Build history of the part. All positions in model axes, mm. Coordinates: 2 decimals unless noted, no trailing zeros. Order: outer loops, then holes, each group sorted by start corner. A loop starts at its lowest first (then second) coordinate and runs counter-clockwise, first axis right, second up. Notation, with made-up numbers: M -9.5,6.25 L 5.5,6.25 A20 ccw 5.5,41.25 Z; hole C 87.5,31.25 d6. An arc over 180 degrees is marked long. Use a Markdown table: item, result. Add a question column.
from build123d import *

# Parameters (mm, degrees)
SKETCH001_R        = 2.05
POCKET_DEPTH       = 96.06142
POLARPATTERN_COUNT = 6


with BuildPart() as part:
    # Sketch → Revolution (revolve)
    with BuildSketch(Plane.XY):
        with BuildLine():
            Line((-2.05, 2.5), (-2.05, -2.5))
            Line((-2.05, -2.5), (-16, -2.5))
            Line((-16, -2.5), (-16, -1.5))
            ThreePointArc((-16, -1.5), (-14.5, 0), (-16, 1.5))
            Line((-16, 1.5), (-16, 2.5))
            Line((-16, 2.5), (-2.05, 2.5))
        make_face()
    revolve(axis=Axis((0, 0, 0), (0, 1, 0)))

    # Sketch001 → Pocket (cut, through all)
    with BuildSketch(Plane.XZ.offset(2.5)):
        with Locations((0, 10)):
            Circle(SKETCH001_R)
    pocket = extrude(amount=-POCKET_DEPTH, mode=Mode.SUBTRACT)

    # PolarPattern: Pocket ×6 about axis
    polarpattern_axis = Axis((0, -2.5, 0), (0, -1, 0))
    for i in range(1, POLARPATTERN_COUNT):
        add(pocket.rotate(polarpattern_axis, i * 360 / POLARPATTERN_COUNT), mode=Mode.SUBTRACT)


solid = part.part
(1) Mould opens along X. For faces 1 (the cylindrical face through (3.47, -1.99, -15.62)), 2 (the cylindrical face through (-8.927, -0.035, -2.967)), 3 (the flat face through (3, -2.5, 0)), 4 (the cylindrical face through (9.76, -0.04, -3.27)) say: released by +X, released by -X, zero draft, split by the parting line, or undercut.
(2) Slice it at C-C on y = 0.3. Give the cut face in (x, z).
(3) Slice it at A-A on z = 0. Give the cut face in (x, y), and give its area (3 significant figures).
(4) Drop flat-ended pins along their axis: P1, Ø3.5, axis at x = 8.66, z = 5, coming from the +Y side; P2, Ø1, axis at y = 0.5, z = -12.5, coming from the +X side; P3, Ø2, axis at y = 1.5, z = -12.5, coming from the -X side; P4, Ø3, axis at x = 0, y = -0.5, coming from the -Z side. Give the stop position or say it passes through.
(5) Drill centre lines: line 1 along Z through (x, y) = (0, 1.8); line 2 along Z through (x, y) = (-0.5, -1.3); line 3 along X through (y, z) = (-1.7, -5.5). Where is each one in solid material? Low to high. Write a range as from..to.
(6) Slice it at B-B on x = 0. Give the cut face in (y, z).
(7) Slice it at D-D on z = 5. State how many separate pieces and enclosed holes the cut face has, and give its area (3 significant figures).
Solutions:
| question | item | result |
|---|---|---|
| 1 | face 1 | split by the parting line |
| 1 | face 2 | undercut |
| 1 | face 3 | zero draft |
| 1 | face 4 | undercut |
| 2 | outline | C 0,0 d29.06; hole C -8.66,-5 d4.1; hole C -8.66,5 d4.1; hole C 0,-10 d4.1; hole C 0,0 d4.1; hole C 0,10 d4.1; hole C 8.66,-5 d4.1; hole C 8.66,5 d4.1 |
| 3 | outline | M -16,-2.5 L -2.05,-2.5 L -2.05,2.5 L -16,2.5 L -16,1.5 A1.5 cw -16,-1.5 Z; M 2.05,-2.5 L 16,-2.5 L 16,-1.5 A1.5 cw 16,1.5 L 16,2.5 L 2.05,2.5 Z |
| 3 | area | 132 mm² |
| 4 | P1 | through |
| 4 | P2 | x = 8.4 |
| 4 | P3 | x = -11.12 |
| 4 | P4 | z = -16 |
| 5 | line 1 | -16..-12.05, -7.95..-2.05, 2.05..7.95, 12.05..16 |
| 5 | line 2 | -15.24..-11.99, -8.01..-1.99, 1.99..8.01, 11.99..15.24 |
| 5 | line 3 | -15.02..-10.65, -6.67..6.67, 10.65..15.02 |
| 6 | outline | M -2.5,-16 L -1.5,-16 A1.5 cw 1.5,-16 L 2.5,-16 L 2.5,-12.05 L -2.5,-12.05 Z; M -2.5,-7.95 L 2.5,-7.95 L 2.5,-2.05 L -2.5,-2.05 Z; M -2.5,2.05 L 2.5,2.05 L 2.5,7.95 L -2.5,7.95 Z; M -2.5,12.05 L 2.5,12.05 L 2.5,16 L 1.5,16 A1.5 cw -1.5,16 L -2.5,16 Z |
| 7 | separate pieces | 3 |
| 7 | enclosed holes | 0 |
| 7 | area | 104 mm² |
